Work out the finished part from the listing and answer in its coordinate system (mm). Coordinates: 2 decimals unless noted, no trailing zeros. Order: outer loops, then holes, each group sorted by start corner. A loop starts at its lowest first (then second) coordinate and runs counter-clockwise, first axis right, second up.
1. The part is cut by section D-D, the plane x = -29. Give the vertices of the cut face in (y, z), then the cut area to 3 significant figures.
2. Flat-ended cylindrical pins translate along their axes: pin 1 Ø1.5 at (x, y) = (1.5, 1.5) entering from -Z; pin 2 Ø1 at (x, y) = (-40.5, 0.5) entering from +Z. Find the tip coordinate at first contact, or state that the pin passes through.
3. The part is cut by section C-C, the plane y = 0.7. Give the vertices of the cut face in (x, z), then the cut area to 3 significant figures.
4. The part is cut by section B-B, the plane z = 0. Give the vertices of the cut face in (x, y), then the cut area to 3 significant figures.
5. Find the intervals of material crossed by probe 1 along X at (y, z) = (1.35, 0); probe 2 along X at (y, z) = (2.35, 0); probe 3 along Z at (x, y) = (37.25, 2.45), in increasing order.
6. The part is cut by section A-A, the plane x = -37.25. Give the vertices of the cut face in (y, z).
```python
from build123d import *

# Parameters (mm, degrees)
SKETCH1_R       = 1.7
SHAPE_DEPTH     = 3
MILL_FILLETS_R  = 1
EDGE_CUTS_DEPTH = 1


with BuildPart() as part:
    # Sketch1 → Shape (new body)
    with BuildSketch(Plane(origin=(0, 0, 0), x_dir=(1, 0, 0), z_dir=(0, 1, 0))):
        with BuildLine():
            Line((-35.329062729, -1.6), (35.329062729, -1.6))
            ThreePointArc((35.329062729, -1.6), (37.25, -2.5), (39.170937271, -1.6))
            Line((39.170937271, -1.6), (40.8, -1.6))
            Line((40.8, -1.6), (40.8, 1.6))
            Line((40.8, 1.6), (39.170937271, 1.6))
            ThreePointArc((39.170937271, 1.6), (37.25, 2.5), (35.329062729, 1.6))
            Line((35.329062729, 1.6), (-35.329062729, 1.6))
            ThreePointArc((-35.329062729, 1.6), (-37.25, 2.5), (-39.170937271, 1.6))
            Line((-39.170937271, 1.6), (-40.8, 1.6))
            Line((-40.8, 1.6), (-40.8, -1.6))
            Line((-40.8, -1.6), (-39.170937271, -1.6))
            ThreePointArc((-39.170937271, -1.6), (-37.25, -2.5), (-35.329062729, -1.6))
        make_face()
        with Locations((37.25, 0)):
            Circle(SKETCH1_R, mode=Mode.SUBTRACT)
        with Locations((-37.25, 0)):
            Circle(SKETCH1_R, mode=Mode.SUBTRACT)
    extrude(amount=SHAPE_DEPTH)

    # Mill fillets
    mill_fillets_edges = [part.edges().sort_by_distance(p)[0] for p in [
        (-35.329062729, 1.5, -1.6),
        (35.329062729, 1.5, -1.6),
        (39.170937271, 1.5, -1.6),
        (39.170937271, 1.5, 1.6),
        (35.329062729, 1.5, 1.6),
        (-35.329062729, 1.5, 1.6),
        (-39.170937271, 1.5, 1.6),
        (-39.170937271, 1.5, -1.6),
    ]]
    fillet(mill_fillets_edges, radius=MILL_FILLETS_R)

    # Sketch2 → Edge cuts (cut)
    with BuildSketch(Plane(origin=(0, 3, 0), x_dir=(1, 0, 0), z_dir=(0, 1, 0))):
        with BuildLine():
            Line((-39.5, -1.60434089), (-39.5, 1.60434089))
            ThreePointArc((-39.5, 1.60434089), (-39.546486866, 1.601085812), (-39.593074903, 1.6))
            Line((-39.593074903, 1.6), (-40.8, 1.6))
            Line((-40.8, 1.6), (-40.8, -1.6))
            Line((-40.8, -1.6), (-39.593074903, -1.6))
            ThreePointArc((-39.593074903, -1.6), (-39.546486866, -1.601085812), (-39.5, -1.60434089))
        make_face()
        with BuildLine():
            ThreePointArc((39.593074903, 1.6), (39.546486866, 1.601085812), (39.5, 1.60434089))
            Line((39.5, 1.60434089), (39.5, -1.60434089))
            ThreePointArc((39.5, -1.60434089), (39.546486866, -1.601085812), (39.593074903, -1.6))
            Line((39.593074903, -1.6), (40.8, -1.6))
            Line((40.8, -1.6), (40.8, 1.6))
            Line((40.8, 1.6), (39.593074903, 1.6))
        make_face()
    extrude(amount=-EDGE_CUTS_DEPTH, mode=Mode.SUBTRACT)


solid = part.part
```
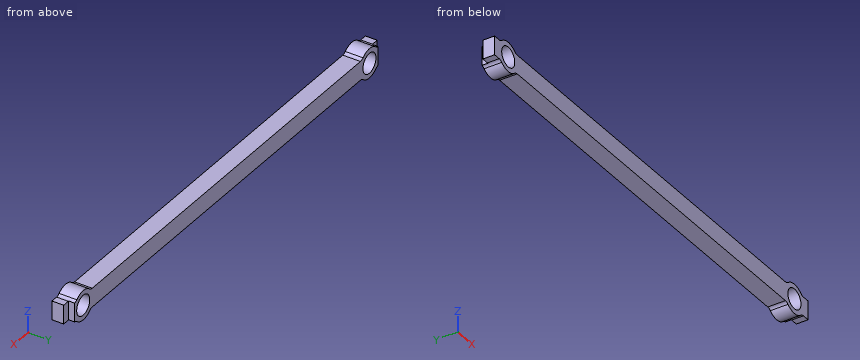
Geometry says:
1. outline: (0, -1.6) - (3, -1.6) - (3, 1.6) - (0, 1.6) - close
1. area: 9.60 mm2
2. pin 1: stops at z = -1.6
2. pin 2: stops at z = 1.6
3. outline: (-40.8, -1.6) - (-39.59, -1.6) arc R1 cw to (-38.92, -1.86) arc R2.5 ccw to (-35.58, -1.86) arc R1 cw to (-34.91, -1.6) - (34.91, -1.6) arc R1 cw to (35.58, -1.86) arc R2.5 ccw to (38.92, -1.86) arc R1 cw to (39.59, -1.6) - (40.8, -1.6) - (40.8, 1.6) - (39.59, 1.6) arc R1 cw to (38.92, 1.86) arc R2.5 ccw to (35.58, 1.86) arc R1 cw to (34.91, 1.6) - (-34.91, 1.6) arc R1 cw to (-35.58, 1.86) arc R2.5 ccw to (-38.92, 1.86) arc R1 cw to (-39.59, 1.6) - (-40.8, 1.6) - close; hole circle Ø3.4 at (-37.25, 0); hole circle Ø3.4 at (37.25, 0)
3. area: 253 mm2
4. outline: (-40.8, 0) - (-38.95, 0) - (-38.95, 3) - (-39.5, 3) - (-39.5, 2) - (-40.8, 2) - close; (-35.55, 0) - (35.55, 0) - (35.55, 3) - (-35.55, 3) - close; (38.95, 0) - (40.8, 0) - (40.8, 2) - (39.5, 2) - (39.5, 3) - (38.95, 3) - close
4. area: 222 mm2
5. probe 1: x = -40.8 to -38.95, -35.55 to 35.55, 38.95 to 40.8
5. probe 2: x = -39.5 to -38.95, -35.55 to 35.55, 38.95 to 39.5
5. probe 3: z = -2.5 to -1.7, 1.7 to 2.5
6. outline: (0, -2.5) - (3, -2.5) - (3, -1.7) - (0, -1.7) - close; (0, 1.7) - (3, 1.7) - (3, 2.5) - (0, 2.5) - close
